Source: CAD feature listing. Evaluate the final solid. Frame: model axes, mm. Give positions to 0.01 mm unless a question says otherwise; leave off trailing zeros. Order: outer loops, then holes, each group sorted by start corner. A loop starts at its lowest first (then second) coordinate and runs counter-clockwise, first axis right, second up.
from build123d import *

# Parameters (mm, degrees)
EXTRUDE_485_DEPTH         = 4
CUT_EXTRUDE_M5_DEPTH      = 8.495721002
CUT_EXTRUDE_M5_DEPTH_BACK = 8.495721002
SKETCH_527_R              = 2.5


with BuildPart() as part:
    # Sketch 341 → Extrude 485 (new body)
    with BuildSketch(Plane.XY):
        Polygon((4.792007234, 0), (2.396003617, 4.15), (-2.396003617, 4.15), (-4.792007234, 0), (-2.396003617, -4.15), (2.396003617, -4.15), align=None)
    extrude(amount=EXTRUDE_485_DEPTH)

    # Sketch 527 → Отверстие_под_M5 (cut, two sides: drawn at the far end of the back side and taken through both)
    with BuildSketch(Plane.XY.offset(-CUT_EXTRUDE_M5_DEPTH_BACK)):
        Circle(SKETCH_527_R)
    extrude(amount=CUT_EXTRUDE_M5_DEPTH + CUT_EXTRUDE_M5_DEPTH_BACK, mode=Mode.SUBTRACT)


solid = part.part
1) Section query B-B on z = 2.2. Output: boundary loops of the cut face in (x, y).
Checks:
outline: (-4.79, 0) - (-2.4, -4.15) - (2.4, -4.15) - (4.79, 0) - (2.4, 4.15) - (-2.4, 4.15) - close; hole circle Ø5 at (0, 0)
2) Pull-direction query (Y, two-part tool) for faces 1 (the face through (0, 4.15, 2)), 2 (the face through (3.58, -2.1, 1.97)), 3 (the face through (-0.54, -2.44, 1.97)); classes: +Y half, -Y half, draft (parallel to the pull), parting line (faces both ways), or undercut.
Checks:
face 1: +Y half
face 2: -Y half
face 3: undercut
3) Section query C-C on y = -1. Output: boundary loops of the cut face in (x, z), and give its area (3 significant figures).
Checks:
outline: (-4.21, 0) - (-2.29, 0) - (-2.29, 4) - (-4.21, 4) - close; (2.29, 0) - (4.21, 0) - (4.21, 4) - (2.29, 4) - close
area: 15.4 mm2
4) Section query D-D on x = 3.5. Output: boundary loops of the cut face in (y, z).
Checks:
outline: (-2.24, 0) - (2.24, 0) - (2.24, 4) - (-2.24, 4) - close
5) Ray query, L1, parallel to Y at x = 0, z = 0.3; L2, parallel to Y at x = -2, z = 3.85; L3, parallel to X at y = -0.75, z = 2.95. Return the intervals inside material, ascending.
Checks:
L1: y = -4.15 to -2.5, 2.5 to 4.15
L2: y = -4.15 to -1.5, 1.5 to 4.15
L3: x = -4.36 to -2.38, 2.38 to 4.36
6) Section query A-A on x = 2. Output: boundary loops of the cut face in (y, z).
Checks:
outline: (-4.15, 0) - (-1.5, 0) - (-1.5, 4) - (-4.15, 4) - close; (1.5, 0) - (4.15, 0) - (4.15, 4) - (1.5, 4) - close
